Can you work these out from the drawing? Everything is in mm from the part's minimum corner. A direction names the side the tool comes from. Coordinates: 2 decimals unless noted, no trailing zeros. Loops run counter-clockwise (first coordinate to the right, second up) from the corner with the lowest first, then second, coordinate; pieces in that order, holes last. Notation, with made-up numbers: (85, 83) -> (132, 83) arc R16 cw to (132, 97) -> close; hole circle Ø5 at (73, 3). An arc over 180 degrees is marked (long way). Put each result on its own line as item: value. Start each with the question number.
Item 1: If we section it at C-C on y = 2.95: Please give me the cut outline in (x, z), plus the area to 3 significant figures.
Item 2: We'd pull the mould along X, two halves only. Please class the marked faces 3 and 4: pulls with the +X half, pulls with the -X half, needs draft (parallel to the pull), parting line crosses it, or undercut.
Item 3: If we section it at D-D on z = 16: Please give me the cut outline in (x, y), plus the area to 3 significant figures.
Item 4: For the marked faces 1 and 2, which set-ups out of +Z, -Z, +X, -X, +Y, -Y let a thin tool reach every point of the face, with its end or its side?
Item 5: If we section it at B-B on x = 24: Please give me the cut outline in (y, z).
Item 6: Will these pins go through, and if not, where does the flat tip stop? P1, Ø2, axis at x = 24, z = 25.5, coming from the +Y side; P2, Ø1, axis at y = 1.5, z = 11.5, coming from the -X side; P3, Ø2, axis at y = 3, z = 40, coming from the +X side.
Item 7: Please list where these lines run through material, in increasing order: L1, parallel to Z at x = 21, y = 2; L2, parallel to X at y = 3.15, z = 24; L3, parallel to Y at x = 34, z = 9.5. Write a range as from..to.
Item 8: If we section it at A-A on z = 24: Please give me the cut outline in (x, y), plus the area to 3 significant figures.
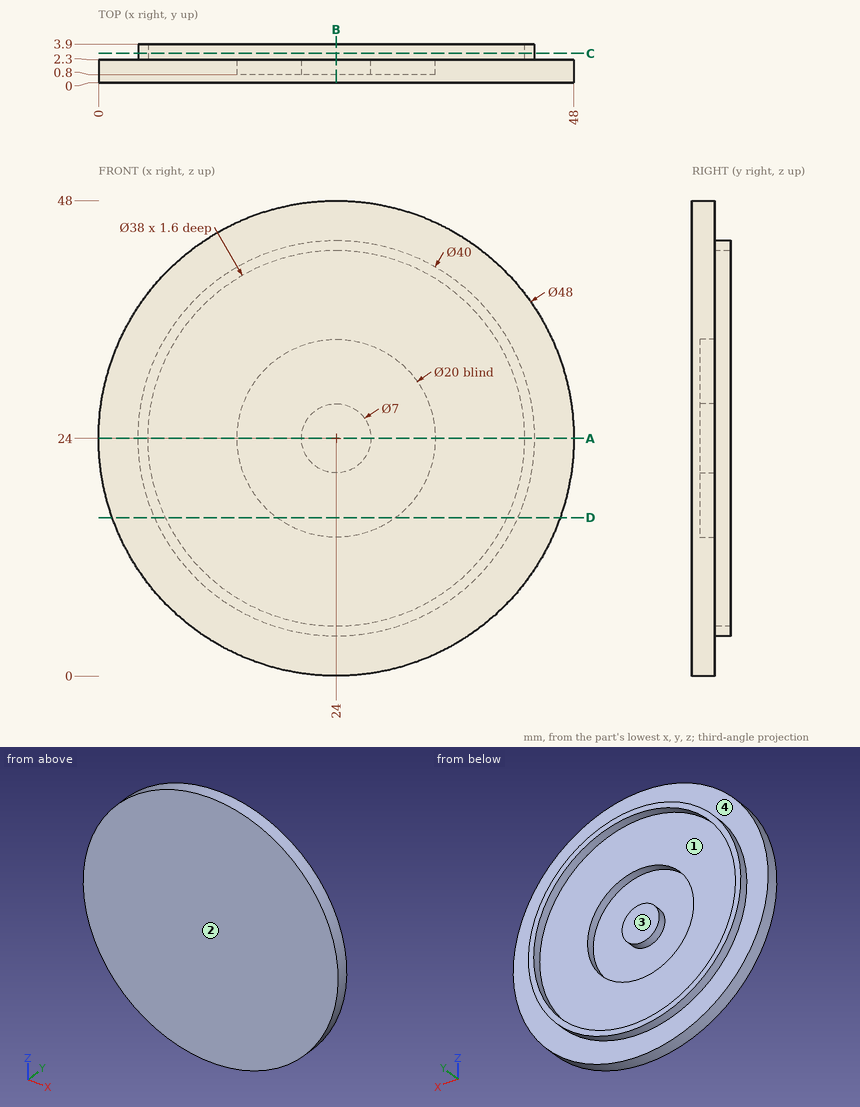
Solutions:
1. outline: circle Ø40 at (24, 24); hole circle Ø38 at (24, 24)
1. area: 123 mm^2
2. face 3: undercut
2. face 4: needs draft
3. outline: (1.37, 0) -> (46.63, 0) -> (46.63, 2.3) -> (42.33, 2.3) -> (42.33, 3.9) -> (41.23, 3.9) -> (41.23, 2.3) -> (30, 2.3) -> (30, 0.8) -> (18, 0.8) -> (18, 2.3) -> (6.77, 2.3) -> (6.77, 3.9) -> (5.67, 3.9) -> (5.67, 2.3) -> (1.37, 2.3) -> close
3. area: 89.6 mm^2
4. face 1: +Y
4. face 2: +Z, -Z, +X, -X, -Y
5. outline: (0, 0) -> (2.3, 0) -> (2.3, 4) -> (3.9, 4) -> (3.9, 5) -> (2.3, 5) -> (2.3, 14) -> (0.8, 14) -> (0.8, 20.5) -> (2.3, 20.5) -> (2.3, 27.5) -> (0.8, 27.5) -> (0.8, 34) -> (2.3, 34) -> (2.3, 43) -> (3.9, 43) -> (3.9, 44) -> (2.3, 44) -> (2.3, 48) -> (0, 48) -> close
6. P1: y = 2.3
6. P2: x = 3.22
6. P3: x = 42.5
7. L1: 0.19..14.46, 22.2..25.8, 33.54..47.81
7. L2: 4..5, 43..44
7. L3: 0..2.3
8. outline: (0, 0) -> (48, 0) -> (48, 2.3) -> (44, 2.3) -> (44, 3.9) -> (43, 3.9) -> (43, 2.3) -> (34, 2.3) -> (34, 0.8) -> (27.5, 0.8) -> (27.5, 2.3) -> (20.5, 2.3) -> (20.5, 0.8) -> (14, 0.8) -> (14, 2.3) -> (5, 2.3) -> (5, 3.9) -> (4, 3.9) -> (4, 2.3) -> (0, 2.3) -> close
8. area: 94.1 mm^2
